Autodesk Inventor part; units mm, degrees
ref_plane "YZ Plane" through (0, 0, 0) normal (1, 0, 0) x (0, 1, 0)
ref_plane "XZ Plane" through (0, 0, 0) normal (0, 1, 0) x (-1, 0, 0)
ref_plane "XY Plane" through (0, 0, 0) normal (0, 0, 1) x (1, 0, 0)
sketch "草图2" plane through (0, 0, 0) normal (0, 0, 1) x (1, 0, 0)
  line L0 (4.3301, -7.5) -> (-4.3301, -7.5)
  line L1 (-4.3301, -7.5) -> (-8.6603, 0)
  line L2 (-8.6603, 0) -> (-4.3301, 7.5)
  line L3 (-4.3301, 7.5) -> (4.3301, 7.5)
  line L4 (4.3301, 7.5) -> (8.6603, 0)
  line L5 (8.6603, 0) -> (4.3301, -7.5)
  line L6 (0, 0) -> (0, 3.4444)
  circle A0 centre (0, 0) radius 4
  point P0 (0, 7.5)
  dimension "d6" = 3.4444
  dimension "d7" = 15
  dimension "d8" = 8
extrude "拉伸2" add sketch "草图2" along normal blind 6
thread "螺纹1"
sketch "草图3" plane through (0, 0, 6) normal (0, 0, 1) x (1, 0, 0)
  line L0 (-4.3301, -7.5) -> (4.3301, -7.5)
  line L1 (-1, 7.5) -> (1, 7.5)
  line L2 (1, 7.5) -> (1, -7.5)
  line L3 (1, -7.5) -> (-1, -7.5)
  line L4 (-1, -7.5) -> (-1, 7.5)
  point P0 (0, 0)
  dimension "d13" = 2
  dimension "d14" = 1
  dimension "d15" = 15
extrude "拉伸3" cut sketch "草图3" against normal blind 2
pattern_circular "环形阵列1" count 3 over 360 about axis through (0, 0, -10) along (0, 0, 1) of "拉伸3"
properties part number "砂轮架固定销螺丝"
Work out the finished part from the listing and answer in its coordinate system (mm). A direction names the side the tool comes from. Give positions to 0.01 mm unless a question says otherwise; leave off trailing zeros. Order: outer loops, then holes, each group sorted by start corner. A loop starts at its lowest first (then second) coordinate and runs counter-clockwise, first axis right, second up. Notation, with made-up numbers: (-6, 78.25) - (42, 78.25) arc R12 cw to (42, 82.25) - close; hole circle Ø11 at (63, -29.5). An arc over 180 degrees is marked (long way). One line per item, written item: value. Start each with the question number.
1. Each of these flat-tipped pins is pushed along its axis until it touches: pin 1 Ø1 at (y, z) = (5.5, 5) entering from +X; pin 2 Ø1.6 at (x, y) = (0, -5) entering from +Z; pin 3 Ø0.6 at (y, z) = (-6, 5) entering from -X. Where does it stop, or does it pass through?
2. Section B-B, the plane y = -3.5 is taken. Write down the section's boundary in (x, z), then the cut area to 3 significant figures.
3. Which of the six approach directions +Z, -Z, +X, -X, +Y, -Y give full straight-line access (tool end or side, diameter ignored) to faces 1 (the face through (-5.403, 1.965, 5.014)), 2 (the face through (1, -6, 5)), 3 (the face through (1.846, 3.549, 2.291))?
4. Section C-C, the plane z = 3.35 is taken. Write down the section's boundary in (x, y), then the cut area to 3 significant figures.
5. Section A-A, the plane x = 0 is taken. Write down the section's boundary in (y, z), then the cut area to 3 significant figures.
6. For a pull along X with two mould halves and no side action, classify faces 4 (the face through (-1, 6, 5)), 5 (the face through (6, 0, 6)), 6 (the face through (6.526, -3.698, 2.958)) as released by +X, released by -X, zero draft, split by the parting line, or undercut.
7. Section D-D, the plane z = 4.65 is taken. Count the separate pieces of the cut face and the enclosed holes in it, then the cut area to 3 significant figures.
8. Consider line 1 (Y direction, x = 0, z = 2.35); line 2 (Y direction, x = 1.25, z = 2.1); line 3 (X direction, y = 3.25, z = 4.35). Determine where each line is inside the solid, lowest interval first.
Filled sheet:
1. pin 1: x = 5.77
1. pin 2: z = 4
1. pin 3: x = -5.37
2. outline: (-6.64, 0) - (-1.94, 0) - (-1.94, 6) - (-4.06, 6) - (-4.06, 4) - (-6.64, 4) - close; (1.94, 0) - (6.64, 0) - (6.64, 4) - (4.06, 4) - (4.06, 6) - (1.94, 6) - close
2. area: 46.1 mm²
3. face 1: +Z
3. face 2: +Z, +Y, -Y
3. face 3: +Z, -Z
4. outline: (-8.66, 0) - (-4.33, -7.5) - (4.33, -7.5) - (8.66, 0) - (4.33, 7.5) - (-4.33, 7.5) - close; hole circle Ø8 at (0, 0)
4. area: 145 mm²
5. outline: (-7.5, 0) - (-4, 0) - (-4, 4) - (-7.5, 4) - close; (4, 0) - (7.5, 0) - (7.5, 4) - (4, 4) - close
5. area: 28.0 mm²
6. face 4: undercut
6. face 5: zero draft
6. face 6: released by +X
7. separate pieces: 6
7. enclosed holes: 0
7. area: 102 mm²
8. line 1: -7.5 to -4, 4 to 7.5
8. line 2: -7.5 to -3.8, 3.8 to 7.5
8. line 3: -3.63 to -2.33, 2.33 to 3.63
